Can you work these out from the model? Positions are in its coordinate system, mm. Face numbers are marked on the shaded views. Coordinates: 2 decimals unless noted, no trailing zeros. Order: outer loops, then holes, each group sorted by start corner. A loop starts at its lowest first (then second) coordinate and runs counter-clockwise, first axis right, second up. Notation, with made-up numbers: (11.5, 27.5) -> (37.5, 27.5) arc R26 ccw to (37.5, 66.5) -> close; hole circle Ø1 at (72.5, 30.25). An arc over 180 degrees is marked (long way). Use a Markdown table: item, result. Add a question column.
1. If I drill on line 1 along X through (y, z) = (40, 1.95); line 2 along Z through (x, y) = (23, 32); line 3 along X through (y, z) = (75, 1.85), over which ranges is the centre line in solid material (lowest first)? Write a range as from..to.
2. We'd pull the mould along Z, two halves only. Please class the marked faces 1, 2, 3 and 4: pulls with the +Z half, pulls with the -Z half, needs draft (parallel to the pull), parting line crosses it, or undercut.
3. Suppose I cut it at D-D, the plane y = 30. List the corners of the cut face in (x, z) for me.
4. Suppose I cut it at B-B, the plane y = 40. List the corners of the cut face in (x, z) for me.
5. For pin 1 Ø5 at (x, y) = (24, 75) entering from -Z; pin 2 Ø6 at (x, z) = (45.5, 24.5) entering from +Y; pin 3 Ø2.5 at (x, z) = (44, 56) entering from +Y; pin 4 Ø5 at (x, y) = (6, 50) entering from +Z, each with a flat end and sliding along its axis, tell me the tip position at first contact or that it passes through.
6. Suppose I cut it at A-A, the plane x = 9.5. List the corners of the cut face in (y, z) for me, then the cut area to 3 significant figures.
7. Suppose I cut it at C-C, the plane x = 56. List the corners of the cut face in (y, z) for me, then the cut area to 3 significant figures.
Autodesk Inventor part; units mm, degrees
ref_plane "YZ Plane" through (0, 0, 0) normal (1, 0, 0) x (0, 1, 0)
ref_plane "XZ Plane" through (0, 0, 0) normal (0, 1, 0) x (-1, 0, 0)
ref_plane "XY Plane" through (0, 0, 0) normal (0, 0, 1) x (1, 0, 0)
sketch "Szkic1" plane through (0, 0, 0) normal (0, 0, 1) x (1, 0, 0)
  line L0 (0, 80) -> (62, 80)
  line L1 (62, 80) -> (62, 0)
  line L2 (62, 0) -> (0, 0)
  line L3 (0, 0) -> (0, 80)
  point P0 (0, 0)
  dimension "d0" = 80
  dimension "d1" = 62
extrude "Wyciągnięcie proste1" add sketch "Szkic1" along normal blind 3
sketch "Szkic2" plane through (0, 0, 3) normal (0, 0, 1) x (1, 0, 0)
  line L0 (0, 80) -> (0, 0)
  line L1 (62, 80) -> (0, 80)
  line L2 (31, 80) -> (31, 0) construction
  line L3 (0, 0) -> (62, 0)
  line L4 (56, 75) -> (56, 50) construction
  line L5 (56, 62.5) -> (62, 62.5) construction
  line L6 (40, 30) -> (40, 5) construction
  line L7 (40, 17.5) -> (62.4441, 17.5) construction
  point P0 (6, 75)
  point P1 (24, 75)
  point P2 (24, 50)
  point P3 (6, 50)
  point P4 (38, 50)
  point P5 (38, 75)
  point P6 (22, 30)
  point P7 (22, 5)
  dimension "d4" = 18
  dimension "d5" = 25
  dimension "d6" = 6
  dimension "d7" = 5
  dimension "d10" = 32
  dimension "d15" = 18
  dimension "d16" = 25
  dimension "d17" = 45
hole "Otwór1" at (6, 75, 3) at (24, 75, 3) at (24, 50, 3) at (6, 50, 3) at (38, 50, 3) at (56, 50, 3) at (56, 75, 3) at (38, 75, 3) at (22, 30, 3) at (40, 30, 3) at (40, 5, 3) at (22, 5, 3) direction (0, 0, -1) diameter 4 end through all
sketch "Szkic3" plane through (0, 0, 0) normal (0, -1, 0) x (1, 0, 0)
  line L0 (0, 0) -> (62, 0)
  line L1 (62, 0) -> (62, 55)
  line L2 (62, 55) -> (0, 55)
  line L3 (0, 55) -> (0, 0)
  line L4 (62, 0) -> (62, 3)
  point P0 (62, 1.5)
  dimension "d25" = 55
extrude "Wyciągnięcie proste2" add sketch "Szkic3" along normal blind 3
sketch "Szkic4" plane through (0, 0, 55) normal (0, 0, 1) x (1, 0, 0)
  line L0 (62, 80) -> (62, -3)
  line L1 (62, -3) -> (0, -3)
  line L2 (0, -3) -> (0, 44)
  line L3 (0, 44) -> (62, 44)
  line L4 (62, 44) -> (62, -3)
  line L5 (0, 0) -> (0, -3)
  point P0 (0, -1.5)
  dimension "d28" = 47
extrude "Wyciągnięcie proste3" add sketch "Szkic4" along normal blind 3
sketch "Szkic5" plane through (0, 0, 0) normal (0, 0, -1) x (-1, 0, 0)
  line L0 (0, -3) -> (-62, -3)
  line L1 (0, -3) -> (0, 80)
  line L2 (-31, -3) -> (-31, 80) construction
  line L3 (-62, 80) -> (0, 80)
  point P0 (0, 0)
  point P1 (-6, 40)
  point P2 (-56, 40)
  dimension "d31" = 43
  dimension "d32" = 6
hole "Otwór2" at (6, 40, 0) at (56, 40, 0) direction (0, 0, 1) diameter 4 end up to surface
thread "Gwint1"
thread "Gwint2"
thread "Gwint3"
thread "Gwint4"
thread "Gwint5"
thread "Gwint6"
thread "Gwint7"
thread "Gwint8"
thread "Gwint9"
thread "Gwint10"
thread "Gwint11"
thread "Gwint12"
thread "Gwint13"
thread "Gwint14"
sketch "Szkic6" plane through (0, 0, 0) normal (0, 1, 0) x (1, 0, 0)
  line L0 (0, -18) -> (19, -18)
  line L1 (19, -18) -> (19, -26)
  line L2 (19, -26) -> (0, -26)
  line L3 (0, -26) -> (0, -18)
  line L4 (62, -3) -> (0, -3)
  point P0 (0, 0)
  dimension "d68" = 15
  dimension "d69" = 8
  dimension "d70" = 19
extrude "Wyciągnięcie proste4" cut sketch "Szkic6" against normal through all
full round fillet "Zaokrąglenie1" first side at (6.3333, -1, 18) centre faces at (19, -1, 20.6667) second side at (6.3333, -2, 26)
sketch "Szkic7" plane through (0, -3, 0) normal (0, -1, 0) x (1, 0, 0)
  line L0 (0, 58) -> (62, 58)
  line L1 (0, 26) -> (0, 58)
  point P0 (0, 0)
  point P1 (15, 40)
  dimension "d73" = 18
  dimension "d74" = 15
hole "Otwór3" at (15, -3, 40) direction (0, 1, 0) diameter 4 end through all
fillet "Zaokrąglenie2" radius 2 2 edges at (31, -3, 58) (31, -3, 0)
sketch "Szkic8" plane through (0, 0, 58) normal (0, 0, 1) x (1, 0, 0)
  line L0 (62, 44) -> (0, 44)
  line L1 (31, 44) -> (31, 0) construction
  line L2 (62, 0) -> (0, 0)
  line L3 (0, 80) -> (0, 0)
  point P0 (9.5, 40)
  point P1 (52.5, 2)
  dimension "d83" = 43
  dimension "d84" = 38
  dimension "d85" = 21.5
  dimension "d86" = 4
hole "Otwór4" at (9.5, 40, 58) at (52.5, 2, 58) direction (0, 0, -1) diameter 3 depth 8 tip angle 118
properties part number "gantry"
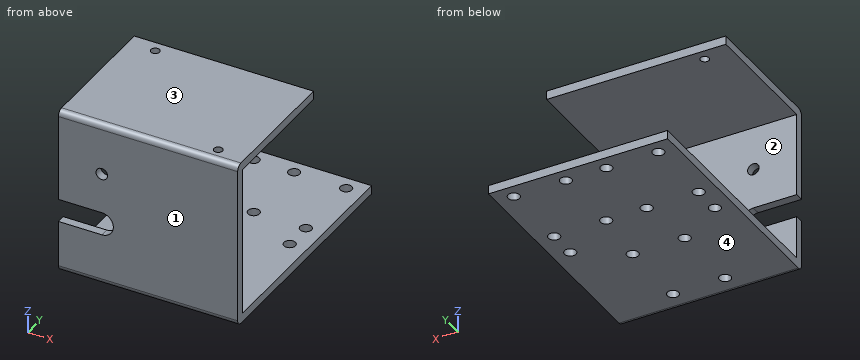
Worked out:
| question | item | result |
|---|---|---|
| 1 | line 1 | x = 0..4, 8..54, 58..62 |
| 1 | line 2 | z = 0..3, 55..58 |
| 1 | line 3 | x = 0..4, 8..22, 26..36, 40..54, 58..62 |
| 2 | face 1 | needs draft |
| 2 | face 2 | undercut |
| 2 | face 3 | pulls with the +Z half |
| 2 | face 4 | pulls with the -Z half |
| 3 | outline | (0, 0) -> (20, 0) -> (20, 3) -> (0, 3) -> close; (0, 55) -> (62, 55) -> (62, 58) -> (0, 58) -> close; (24, 0) -> (38, 0) -> (38, 3) -> (24, 3) -> close; (42, 0) -> (62, 0) -> (62, 3) -> (42, 3) -> close |
| 4 | outline | (0, 0) -> (4, 0) -> (4, 3) -> (0, 3) -> close; (0, 55) -> (8, 55) -> (8, 58) -> (0, 58) -> close; (8, 0) -> (54, 0) -> (54, 3) -> (8, 3) -> close; (11, 55) -> (62, 55) -> (62, 58) -> (11, 58) -> close; (58, 0) -> (62, 0) -> (62, 3) -> (58, 3) -> close |
| 5 | pin 1 | stops at z = 0 |
| 5 | pin 2 | stops at y = 0 |
| 5 | pin 3 | stops at y = 44 |
| 5 | pin 4 | stops at z = 3 |
| 6 | outline | (-3, 2) arc R2 ccw to (-1, 0) -> (80, 0) -> (80, 3) -> (0, 3) -> (0, 18) -> (-3, 18) -> close; (-3, 26) -> (0, 26) -> (0, 55) -> (38.5, 55) -> (38.5, 58) -> (-1, 58) arc R2 ccw to (-3, 56) -> close; (41.5, 55) -> (44, 55) -> (44, 58) -> (41.5, 58) -> close |
| 6 | area | 511 mm² |
| 7 | outline | (-3, 2) arc R2 ccw to (-1, 0) -> (38, 0) -> (38, 3) -> (0, 3) -> (0, 55) -> (44, 55) -> (44, 58) -> (-1, 58) arc R2 ccw to (-3, 56) -> close; (42, 0) -> (48, 0) -> (48, 3) -> (42, 3) -> close; (52, 0) -> (73, 0) -> (73, 3) -> (52, 3) -> close; (77, 0) -> (80, 0) -> (80, 3) -> (77, 3) -> close |
| 7 | area | 508 mm² |
